```python
from build123d import *


with BuildPart() as part:
    # Sketch1 → Revolve1 (revolve)
    with BuildSketch(Plane.XY):
        Polygon((-4.8895, 0), (-4.8895, -3.048), (-6.35, -3.048), (-6.35, -1.524), (-9.525, -1.524), (-9.525, -0.762), (-8.763, 0), align=None)
    revolve(axis=Axis((0, 0, 0), (0, -1, 0)))


solid = part.part
```
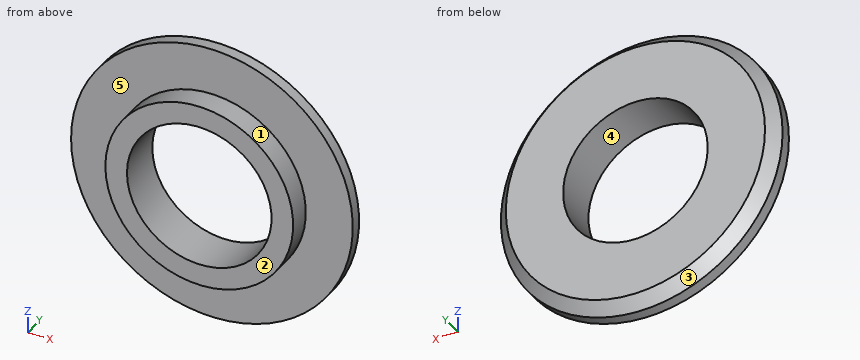
Design review of the part built by this model. Coordinates are the model's own, in mm. Face numbers are marked on the shaded views. A direction names the side the tool comes from. Coordinates: 2 decimals unless noted, no trailing zeros.
1) Mouldability with a two-part tool opening along Z and no side actions: class the marked faces 3, 4 and 5 as +Z half, -Z half, draft (parallel to the pull), parting line (faces both ways), or undercut.
2) Machinability: for the marked faces 1 and 2, which of the approach directions +Z, -Z, +X, -X, +Y, -Y give a long, thin tool a straight path to every point of the face, cutting with its end or side? Answer none if there is none.
3) Insertion check: pin 1 (2 mm diameter, centred on x = 7, z = 7, fed in from -Y); pin 2 (1.5 mm diameter, centred on x = 5, y = -2.5, fed in from +Z). Each pin has a flat end and moves straight along its axis. Give the tip position at first contact, or say it passes through.
4) To check wall thickness, follow L1, parallel to Z at x = 0, y = -1 (1 decimal); L2, parallel to X at y = -2.2, z = 0. State the ranges of each line that lie inside material, in increasing order.
Check result:
1. face 3: parting line
1. face 4: undercut
1. face 5: draft
2. face 1: -Y
2. face 2: +Z, -Z, +X, -X, -Y
3. pin 1: stops at y = -1.52
3. pin 2: stops at z = 4.72
4. L1: z = -9.5 to -4.9, 4.9 to 9.5
4. L2: x = -6.35 to -4.89, 4.89 to 6.35
